Here's how the part is built. I have some questions about the finished solid (model axes, mm). Round coordinates to 2 decimals unless told otherwise and drop trailing zeros. Loops run counter-clockwise (first coordinate to the right, second up) from the corner with the lowest first, then second, coordinate; pieces in that order, holes last. Notation, with made-up numbers: (43.25, 26.5) - (97.25, 26.5) arc R25 ccw to (97.25, 58.5) - close; hole circle Ø8 at (68, 43). An arc over 180 degrees is marked (long way). Answer as a JSON object with one key per item and string values. Group by question number.
1) I want a section at B-B, the plane z = 9. Please give me the cut outline in (x, y), then the cut area to 3 significant figures.
2) I want a section at A-A, the plane x = -6.5. Please give me the cut outline in (y, z), then the cut area to 3 significant figures.
3) Will these pins go through, and if not, where does the flat tip stop? P1, Ø1.4, axis at x = 1, y = -3, coming from the -Z side; P2, Ø4, axis at y = -6, z = -29.5, coming from the +X side; P3, Ø1.4, axis at x = 1, y = -3.5, coming from the +Z side.
4) If I drill on line 1 along X through (y, z) = (-3.75, -10); line 2 along Z through (x, y) = (-7.5, -0.25); line 3 along Z through (x, y) = (-3.5, -5.5), over which ranges is the centre line in solid material (lowest first)? Write a range as [from, to].
from build123d import *

# Parameters (mm, degrees)
F0_W     = 67.056
F0_H     = 138.176
F1_DEPTH = 6.858
F2_R     = 12.7
F3_R     = 12.7
F4_R     = 12.7
F5_R     = 12.7
F8_W     = 2.7374484343
F8_H     = 9.4099827111
F9_DEPTH = 1.27
F10_R    = 0.635
F11_R    = 0.635
F12_R    = 0.635
F13_R    = 0.635


# Not quite as in the source:
# - the program builds the solid bodies; features that only make, move or delete a surface that nothing else refers to are left out


with BuildPart() as f1:
    # F0 (on Front) → F1 (new body)
    with BuildSketch(Plane.XZ):
        with Locations((-33.528, 1.5209056576)):
            Rectangle(F0_W, F0_H)
    extrude(amount=F1_DEPTH)

    # F2
    f2_edges = [f1.edges().sort_by_distance(p)[0] for p in [
        (-67.056, -3.429, 70.608906),
    ]]
    fillet(f2_edges, radius=F2_R)

    # F3
    f3_edges = [f1.edges().sort_by_distance(p)[0] for p in [
        (0, -3.429, 70.608906),
    ]]
    fillet(f3_edges, radius=F3_R)

    # F4
    f4_edges = [f1.edges().sort_by_distance(p)[0] for p in [
        (-67.056, -3.429, -67.567094),
    ]]
    fillet(f4_edges, radius=F4_R)

    # F5
    f5_edges = [f1.edges().sort_by_distance(p)[0] for p in [
        (0, -3.429, -67.567094),
    ]]
    fillet(f5_edges, radius=F5_R)

    # F8 (on face) → F9 (join)
    with BuildSketch(Plane.YZ):
        with Locations((-3.1723636785, 47.4587213248)):
            Rectangle(F8_W, F8_H)
    extrude(amount=F9_DEPTH)

    # F10
    f10_edges = [f1.edges().sort_by_distance(p)[0] for p in [
        (0.635, -1.803639, 52.163713),
    ]]
    fillet(f10_edges, radius=F10_R)

    # F11
    f11_edges = [f1.edges().sort_by_distance(p)[0] for p in [
        (0.635, -1.803639, 42.75373),
    ]]
    fillet(f11_edges, radius=F11_R)

    # F12
    f12_edges = [f1.edges().sort_by_distance(p)[0] for p in [
        (0.635, -4.541088, 52.163713),
    ]]
    fillet(f12_edges, radius=F12_R)

    # F13
    f13_edges = [f1.edges().sort_by_distance(p)[0] for p in [
        (0.635, -4.541088, 42.75373),
    ]]
    fillet(f13_edges, radius=F13_R)


solid = f1.part
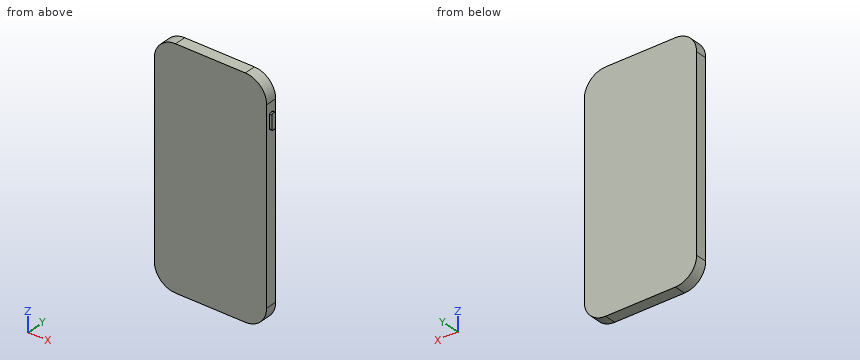
Outcome:
{
 "1": {"outline": "(-67.06, -6.86) - (0, -6.86) - (0, 0) - (-67.06, 0) - close", "area": "460 mm^2"},
 "2": {"outline": "(-6.86, -65.95) - (0, -65.95) - (0, 68.99) - (-6.86, 68.99) - close", "area": "925 mm^2"},
 "3": {"P1": "z = 42.75", "P2": "x = 0", "P3": "z = 52.16"},
 "4": {"line 1": "[-67.06, 0]", "line 2": "[-66.45, 69.5]", "line 3": "[-63.62, 66.66]"}
}
